```python
from build123d import *

# Parameters (mm, degrees)
PAD_DEPTH = 10


with BuildPart() as part:
    # Sketch → Pad (new body)
    with BuildSketch(Plane.XZ):
        with BuildLine():
            Line((0, 0), (0, 15))
            Line((0, 15), (-10, 15))
            Line((-10, 15), (-10, 55))
            Line((-10, 55), (0, 55))
            Line((0, 55), (0, 70))
            Line((0, 70), (80, 70))
            ThreePointArc((85, 65), (83.535534, 68.535534), (80, 70))
            Line((85, 65), (85, 15))
            ThreePointArc((85, 15), (86.464466, 11.464466), (90, 10))
            Line((90, 10), (140, 10))
            ThreePointArc((140, 10), (143.535534, 11.464466), (145, 15))
            Line((145, 15), (145, 65))
            ThreePointArc((150, 70), (146.464466, 68.535534), (145, 65))
            Line((150, 70), (230, 70))
            Line((230, 70), (230, 55))
            Line((230, 55), (240, 55))
            Line((240, 55), (240, 15))
            Line((240, 15), (230, 15))
            Line((230, 15), (230, 0))
            Line((230, 0), (0, 0))
        make_face()
    extrude(amount=PAD_DEPTH)


solid = part.part
```
Geometry check sheet. Reference: the model listing, model coordinates, mm. A direction names the side the tool comes from. Give positions to 0.01 mm unless a question says otherwise; leave off trailing zeros. Write each loop counter-clockwise with the first axis right and the second up, starting at its lowest first coordinate (ties: lowest second). Pieces come first, ordered by that corner, then holes. Notation, with made-up numbers: (9.25, 3) -> (27.25, 3) arc R20 ccw to (27.25, 11) -> close; hole circle Ø7 at (-8, -37.5). An arc over 180 degrees is marked (long way). Use one line per item in the form item = value.
Item 1: Sectioned sample at A-A on z = 32.5. Enter the section's corners in (x, y).
Results list:
outline = (-10, -10) -> (85, -10) -> (85, 0) -> (-10, 0) -> close; (145, -10) -> (240, -10) -> (240, 0) -> (145, 0) -> close
Item 2: Mould release check, pull along X, two halves, no side actions. Record for faces 6 (the flat face through (230, -5, 8)), 7 (the cylindrical face through (84, -5, 68)), 8 (the cylindrical face through (147, -5, 69)), 9 (the flat face through (235, -5, 15)): released by +X, released by -X, zero draft, split by the parting line, or undercut.
Results list:
face_6 = released by +X
face_7 = undercut
face_8 = undercut
face_9 = zero draft
Item 3: Sectioned sample at B-B on y = -2.75. Enter the section's corners in (x, z), plus the area to 3 significant figures.
Results list:
outline = (-10, 15) -> (0, 15) -> (0, 0) -> (230, 0) -> (230, 15) -> (240, 15) -> (240, 55) -> (230, 55) -> (230, 70) -> (150, 70) arc R5 ccw to (145, 65) -> (145, 15) arc R5 cw to (140, 10) -> (90, 10) arc R5 cw to (85, 15) -> (85, 65) arc R5 ccw to (80, 70) -> (0, 70) -> (0, 55) -> (-10, 55) -> close
area = 13,300 mm2
Item 4: Depth check by flat-ended pin: pin 1 Ø3 at (x, y) = (-6.5, -5.5) entering from -Z; pin 2 Ø2 at (x, y) = (20.5, -1) entering from -Z; pin 3 Ø3 at (y, z) = (-5.5, 62.5) entering from -X; pin 4 Ø5 at (x, y) = (109, -6) entering from +Z. Enter the tip coordinate at first touch or a pass-through.
Results list:
pin_1 = 15
pin_2 = 0
pin_3 = 0
pin_4 = 10
Item 5: Sectioned sample at C-C on z = 62. Enter the section's corners in (x, y).
Results list:
outline = (0, -10) -> (85, -10) -> (85, 0) -> (0, 0) -> close; (145, -10) -> (230, -10) -> (230, 0) -> (145, 0) -> close
Item 6: Access from +Z, -Z, +X, -X, +Y, -Y to the whole of each face (thin tool, end or side, straight path). Record for faces 1 (the flat face through (230, -5, 63)), 2 (the flat face through (-5, -5, 55)), 3 (the cylindrical face through (86, -5, 12)), 4 (the flat face through (39, -5, 70)), 5 (the flat face through (-5, -5, 15)).
Results list:
face_1 = +Z, +X, +Y, -Y
face_2 = +Z, -X, +Y, -Y
face_3 = +Z, +Y, -Y
face_4 = +Z, +X, -X, +Y, -Y
face_5 = -Z, -X, +Y, -Y
Item 7: Scan lines: line 1 (X direction, y = -1.5, z = 34.5); line 2 (X direction, y = -7.75, z = 57); line 3 (Z direction, x = 98, y = -1). Record each from-to range of solid material in increasing order.
Results list:
line_1 = -10 to 85, 145 to 240
line_2 = 0 to 85, 145 to 230
line_3 = 0 to 10
Item 8: Sectioned sample at D-D on z = 4.5. Enter the section's corners in (x, y).
Results list:
outline = (0, -10) -> (230, -10) -> (230, 0) -> (0, 0) -> close
